Verification items for the finished model (mm, model axes). A direction names the side the tool comes from. Coordinates: 2 decimals unless noted, no trailing zeros. Order: outer loops, then holes, each group sorted by start corner. A loop starts at its lowest first (then second) coordinate and runs counter-clockwise, first axis right, second up. Notation, with made-up numbers: M 71.5,-28 L 125.5,-28 A16 cw 125.5,-8 Z; hole C -25.5,65.25 d4. An arc over 180 degrees is marked long. Return JSON: item names as keys, results as strings. Group by question number.
Q1. Mould release check, pull along Z, two halves, no side actions. Record for faces 4 (the face through (9.51, -0.86, -18.95)), 5 (the face through (0.95, -0.86, 24.73)), 6 (the face through (-1.9, -1.75, 20.5)): pulls with the +Z half, pulls with the -Z half, needs draft (parallel to the pull), parting line crosses it, or undercut.
Q2. Section check C-C, the plane z = 9.5. Enter the section's corners in (x, y), then the cut area to 3 significant figures.
Q3. Section check D-D, the plane x = 0. Enter the section's corners in (y, z), then the cut area to 3 significant figures.
Q4. Section check B-B, the plane y = -1. Enter the section's corners in (x, z), then the cut area to 3 significant figures.
Q5. Thickness scan on probe 1 along Z at (x, y) = (10.5, -1.3); probe 2 along X at (y, z) = (-0.1, -0.5); probe 3 along X at (y, z) = (-0.8, 18). Record the ranges inside material, lowest first.
Q6. Section check A-A, the plane z = -11. Enter the section's corners in (x, y), then the cut area to 3 significant figures.
Q7. Access from +Z, -Z, +X, -X, +Y, -Y to the whole of each face (thin tool, end or side, straight path). Record for faces 1 (the face through (8.8, -0.86, -20.99)), 2 (the face through (8.314, -0.863, -16.689)), 3 (the face through (-1.9, 0, 20.5)).
from build123d import *

# Parameters (mm, degrees)
F0_R     = 1.25
F1_DEPTH = 1.75


with BuildPart() as f1:
    # F0 (on Front) → F1 (new body)
    with BuildSketch(Plane.XZ):
        with BuildLine():
            Line((8.056176, -19.211338), (9.571292, -22.824392))
            ThreePointArc((9.571292, -22.824392), (0, 24.75), (-9.571292, -22.824392))
            Line((-9.571292, -22.824392), (-8.056176, -19.211338))
            ThreePointArc((-8.056176, -19.211338), (-8.293393, -16.719092), (-10.5, -15.536533))
            Line((-10.5, -15.536533), (-14.45036, -15.536533))
            ThreePointArc((-14.45036, -15.536533), (-15.509779, -15.300961), (-16.369542, -14.638638))
            ThreePointArc((-16.369542, -14.638638), (0, 20.35), (16.369542, -14.638638))
            ThreePointArc((16.369542, -14.638638), (15.509779, -15.300961), (14.45036, -15.536533))
            Line((14.45036, -15.536533), (10.5, -15.536533))
            ThreePointArc((10.5, -15.536533), (8.293393, -16.719092), (8.056176, -19.211338))
        make_face()
        with Locations((-10.5, -18.186533)):
            Circle(F0_R, mode=Mode.SUBTRACT)
        with Locations((10.5, -18.186533)):
            Circle(F0_R, mode=Mode.SUBTRACT)
    extrude(amount=F1_DEPTH)


solid = f1.part
Numbers:
{
 "1": {"face 4": "undercut", "face 5": "parting line crosses it", "face 6": "needs draft"},
 "2": {"outline": "M -22.85,-1.75 L -18.57,-1.75 L -18.57,0 L -22.85,0 Z; M 18.57,-1.75 L 22.85,-1.75 L 22.85,0 L 18.57,0 Z", "area": "15.0 mm2"},
 "3": {"outline": "M -1.75,20.35 L 0,20.35 L 0,24.75 L -1.75,24.75 Z", "area": "7.70 mm2"},
 "4": {"outline": "M -16.37,-14.64 A21.32 cw long 16.37,-14.64 A2.5 cw 14.45,-15.54 L 10.5,-15.54 A2.65 ccw 8.06,-19.21 L 9.57,-22.82 A24.75 ccw long -9.57,-22.82 L -8.06,-19.21 A2.65 ccw -10.5,-15.54 L -14.45,-15.54 A2.5 cw Z; hole C -10.5,-18.19 d2.5; hole C 10.5,-18.19 d2.5", "area": "483 mm2"},
 "5": {"probe 1": "z = -22.41 to -19.44, -16.94 to -15.54, 17.59 to 22.41", "probe 2": "x = -24.74 to -21.32, 21.32 to 24.74", "probe 3": "x = -16.99 to -9.73, 9.73 to 16.99"},
 "6": {"outline": "M -22.17,-1.75 L -18.82,-1.75 L -18.82,0 L -22.17,0 Z; M 18.82,-1.75 L 22.17,-1.75 L 22.17,0 L 18.82,0 Z", "area": "11.7 mm2"},
 "7": {"face 1": "-Z, +Y, -Y", "face 2": "+Y, -Y", "face 3": "+Z, -Z, +X, -X, +Y"}
}
